Check sheet for the modelled part. Datum: model origin and axes. Units: mm. Face numbers are marked on the shaded views. Give positions to 0.01 mm unless a question says otherwise; leave off trailing zeros. Order: outer loops, then holes, each group sorted by start corner. A loop starts at its lowest first (then second) coordinate and runs counter-clockwise, first axis right, second up.
from build123d import *

# Parameters (mm, degrees)
SKETCH1_R           = 2
BOSS_EXTRUDE1_DEPTH = 67
CUT_EXTRUDE1_REACH  = 30.5
CUT_EXTRUDE2_REACH  = 28.5
SKETCH3_W           = 59
SKETCH3_H           = 9.6


with BuildPart() as part:
    # Sketch1 → Boss-Extrude1 (new body)
    with BuildSketch(Plane(origin=(0, 0, 0), x_dir=(0, 0, -1), z_dir=(1, 0, 0))):
        with BuildLine():
            Line((11.9, 1.9), (11.9, 0))
            Line((11.9, 0), (0, 0))
            Line((0, 0), (18.5, 18.5))
            Line((18.5, 18.5), (18.5, 21.5))
            ThreePointArc((18.5, 21.5), (23.5, 26.5), (28.5, 21.5))
            Line((28.5, 21.5), (28.5, 18.5))
            Line((28.5, 18.5), (11.9, 1.9))
        make_face()
        with Locations((23.5, 21.5)):
            Circle(SKETCH1_R, mode=Mode.SUBTRACT)
    extrude(amount=BOSS_EXTRUDE1_DEPTH)

    # Sketch2 → Cut-Extrude1 (cut, up to next)
    with BuildSketch(Plane(origin=(0, 0, -28.5), x_dir=(-1, 0, 0), z_dir=(0, 0, -1)), mode=Mode.PRIVATE) as cut_extrude1_sk1:
        with BuildLine():
            Line((-63, 26.5), (-63, 11.5))
            ThreePointArc((-63, 11.5), (-61.828427125, 8.671572875), (-59, 7.5))
            Line((-59, 7.5), (-8, 7.5))
            ThreePointArc((-8, 7.5), (-5.171572875, 8.671572875), (-4, 11.5))
            Line((-4, 11.5), (-4, 26.5))
            Line((-4, 26.5), (-63, 26.5))
        make_face()
    cut_extrude1_tool1 = extrude(cut_extrude1_sk1.sketch, amount=-CUT_EXTRUDE1_REACH, mode=Mode.PRIVATE) & part.part
    add(cut_extrude1_tool1.solids().sort_by_distance((33.5, 17.053049, -28.5))[0], mode=Mode.SUBTRACT)

    # Sketch3 → Cut-Extrude2 (cut, up to next)
    with BuildSketch(Plane.XZ, mode=Mode.PRIVATE) as cut_extrude2_sk1:
        with Locations((33.5, -16.7)):
            Rectangle(SKETCH3_W, SKETCH3_H)
    cut_extrude2_tool1 = extrude(cut_extrude2_sk1.sketch, amount=-CUT_EXTRUDE2_REACH, mode=Mode.PRIVATE) & part.part
    add(cut_extrude2_tool1.solids().sort_by_distance((33.5, 0, -16.7))[0], mode=Mode.SUBTRACT)


solid = part.part
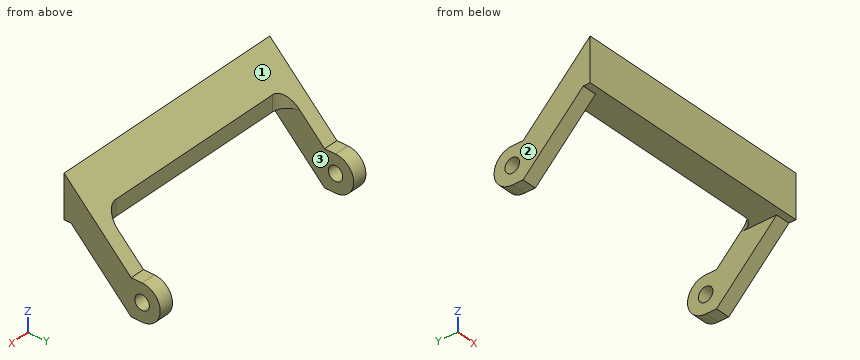
1) Section check C-C, the plane y = 16.75. Record the cut outline in (x, z), then the cut area to 3 significant figures.
Recorded:
outline: (0, -26.75) - (4, -26.75) - (4, -16.75) - (0, -16.75) - close; (63, -26.75) - (67, -26.75) - (67, -16.75) - (63, -16.75) - close
area: 80.0 mm2
2) Section check A-A, the plane z = -23.5. Record the cut outline in (x, y), then the cut area to 3 significant figures.
Recorded:
outline: (0, 13.5) - (4, 13.5) - (4, 19.5) - (0, 19.5) - close; (0, 23.5) - (4, 23.5) - (4, 26.5) - (0, 26.5) - close; (63, 13.5) - (67, 13.5) - (67, 19.5) - (63, 19.5) - close; (63, 23.5) - (67, 23.5) - (67, 26.5) - (63, 26.5) - close
area: 72.0 mm2
3) Draft check along X on the marked faces 1, 2 and 3. Enter one of: +X half, -X half, draft (parallel to the pull), parting line (faces both ways), or undercut.
Recorded:
face 1: draft
face 2: -X half
face 3: undercut
4) Section check B-B, the plane z = -13. Record the cut outline in (x, y).
Recorded:
outline: (0, 3) - (4, 3) - (4, 13) - (0, 13) - close; (63, 3) - (67, 3) - (67, 13) - (63, 13) - close
5) Material ranges on L1, parallel to Z at x = 1.5, y = 21.5; L2, parallel to X at y = 13.25, z = -16.5; L3, parallel to Y at x = 30, z = -8.25, recorded low to high.
Recorded:
L1: z = -28.5 to -25.5, -21.5 to -18.5
L2: x = 0 to 4, 63 to 67
L3: y = 0 to 7.5
6) Depth check by flat-ended pin: pin 1 Ø10 at (x, y) = (27.5, 7) entering from -Z; pin 2 Ø2 at (x, z) = (34.5, -10.5) entering from +Y; pin 3 Ø8 at (y, z) = (5.5, -22) entering from -X; pin 4 Ø0.9 at (x, y) = (64, 19.5) entering from +Z. Enter the tip coordinate at first touch or a pass-through.
Recorded:
pin 1: stops at z = -11.9
pin 2: stops at y = 7.5
pin 3: passes through
pin 4: stops at z = -18.5
7) Section check D-D, the plane y = 5. Record the cut outline in (x, z).
Recorded:
outline: (0, -15) - (4, -15) - (4, -11.9) - (63, -11.9) - (63, -15) - (67, -15) - (67, -5) - (0, -5) - close
